Autodesk Inventor part; units mm, degrees
ref_plane "YZ Plane" through (0, 0, 0) normal (1, 0, 0) x (0, 1, 0)
ref_plane "XZ Plane" through (0, 0, 0) normal (0, 1, 0) x (-1, 0, 0)
ref_plane "XY Plane" through (0, 0, 0) normal (0, 0, 1) x (1, 0, 0)
sketch "Эскиз1" plane through (0, 0, 0) normal (1, 0, 0) x (0, 1, 0)
  circle A0 centre (0, 0) radius 3.5
  dimension "d0" = 7
extrude "Выдавливание1" add sketch "Эскиз1" along normal blind 10
sketch "Эскиз2" plane through (0, 0, 0) normal (-1, 0, 0) x (0, 0, 1)
  circle A0 centre (0, 0) radius 0.6
  dimension "d3" = 1.2
extrude "Выдавливание2" add sketch "Эскиз2" along normal blind 1
sketch "Эскиз3" plane through (10, 0, 0) normal (1, 0, 0) x (0, 0, -1)
  circle A0 centre (0, 0) radius 0.6
  circle A1 centre (0, 0) radius 1.25
  dimension "d6" = 2.5
extrude "Выдавливание3" cut sketch "Эскиз3" against normal blind 8 contours A0 | A1
thread "Резьба1"
properties part number "Bush_Phase" material "Медь"
The listing builds one solid part. Answer for the finished solid, in the listing's coordinates (mm). A direction names the side the tool comes from. Coordinates: 2 decimals unless noted, no trailing zeros. Loops run counter-clockwise (first coordinate to the right, second up) from the corner with the lowest first, then second, coordinate; pieces in that order, holes last. Notation, with made-up numbers: (78, 20.5) -> (107, 20.5) arc R22 ccw to (107, 56.5) -> close; hole circle Ø3 at (78.25, -36.5). An arc over 180 degrees is marked (long way). Write item = value, one per line. Start each with the question number.
1) Straight lines are drawn through the part: line 1 (X direction, y = -1.75, z = -1.75); line 2 (X direction, y = -0.25, z = -0.25); line 3 (Z direction, x = 3.5, y = -0.25). For each, find the intervals that lie inside material, in ascending order. Write a range as from..to.
2) A cutting plane is placed at B-B (x = 0.25). Give the vertices of the cut face in (y, z), then the cut area to 3 significant figures.
3) Given pin 1 Ø3 at (x, z) = (0.5, 2) entering from -Y; pin 2 Ø2 at (x, z) = (2, 2) entering from +Y; pin 3 Ø2 at (x, z) = (8.5, 2.5) entering from +Y; pin 4 Ø4 at (y, z) = (0, 0) entering from +X, each flat-ended and moving along its own axis, determine where each tip first touches the part or whether it passes through.
4) A cutting plane is placed at A-A (z = 0). Give the vertices of the cut face in (x, y).
5) A cutting plane is placed at D-D (y = -1.5). Give the vertices of the cut face in (x, z).
6) A cutting plane is placed at C-C (x = 5.25). Give the vertices of the cut face in (y, z).
7) The mould has two halves that part along Z. Classify faces 1 (the face through (-1, 0, 0)), 2 (the face through (-0.493, -0.506, 0.323)), 3 (the face through (6.06, -1.22, 0.27)): released by +Z, released by -Z, zero draft, split by the parting line, or undercut.
8) A tool of negligible diameter and unlimited length cuts with its end or side. For faces 4 (the face through (4.93, 3.233, 1.341)), 5 (the face through (2, 0, 0)), from which of +Z, -Z, +X, -X, +Y, -Y can it reach the whole face along a straight path? Write none if from no direction.
Responses:
q1.line_1 = 0..10
q1.line_2 = -1..2
q1.line_3 = -3.49..-1.22, 1.22..3.49
q2.outline = circle Ø7 at (0, 0)
q2.area = 38.5 mm²
q3.pin_1 = -3.46
q3.pin_2 = 3.35
q3.pin_3 = 3.16
q3.pin_4 = 10
q4.outline = (-1, -0.6) -> (0, -0.6) -> (0, -3.5) -> (10, -3.5) -> (10, -1.25) -> (2, -1.25) -> (2, 1.25) -> (10, 1.25) -> (10, 3.5) -> (0, 3.5) -> (0, 0.6) -> (-1, 0.6) -> close
q5.outline = (0, -3.16) -> (10, -3.16) -> (10, 3.16) -> (0, 3.16) -> close
q6.outline = circle Ø7 at (0, 0); hole circle Ø2.5 at (0, 0)
q7.face_1 = zero draft
q7.face_2 = split by the parting line
q7.face_3 = undercut
q8.face_4 = +X, -X
q8.face_5 = +X
